Check sheet for the modelled part. Datum: model origin and axes. Units: mm. A direction names the side the tool comes from. Round coordinates to 2 decimals unless told otherwise and drop trailing zeros. Order: outer loops, then holes, each group sorted by start corner. A loop starts at its lowest first (then second) coordinate and runs counter-clockwise, first axis right, second up.
```python
from build123d import *

# Parameters (mm, degrees)
SKETCH2_R           = 4.826
CUT_EXTRUDE1_DEPTH  = 25.4
SKETCH3_W           = 14.986
SKETCH3_H           = 14.986
BOSS_EXTRUDE1_DEPTH = 12.7


with BuildPart() as part:
    # Sketch1 → Revolve1 (revolve)
    with BuildSketch(Plane.XY):
        Polygon((0, 0), (152.4, 0), (152.4, 12.7), (0, 15.875), align=None)
    revolve(axis=Axis((0, 0, 0), (1, 0, 0)))

    # Sketch2 → Cut-Extrude1 (cut)
    with BuildSketch(Plane(origin=(152.4, 0, 0), x_dir=(0, 0, -1), z_dir=(1, 0, 0))):
        Circle(SKETCH2_R)
    extrude(amount=-CUT_EXTRUDE1_DEPTH, mode=Mode.SUBTRACT)

    # Sketch3 → Boss-Extrude1 (add)
    with BuildSketch(Plane.ZY):
        Rectangle(SKETCH3_W, SKETCH3_H)
    extrude(amount=BOSS_EXTRUDE1_DEPTH)


solid = part.part
```
Item 1: Scan lines: line 1 along Y through (x, z) = (135, 0); line 2 along X through (y, z) = (-3, 0); line 3 along X through (y, z) = (-12, 3.5). Record each from-to range of solid material in increasing order.
Answer:
line 1: y = -13.06 to -4.83, 4.83 to 13.06
line 2: x = -12.7 to 127
line 3: x = 0 to 152.4
Item 2: Sectioned sample at C-C (x = 140.5). Record the cut outline in (y, z), and give its area (3 significant figures).
Answer:
outline: circle Ø25.9 at (0, 0); hole circle Ø9.65 at (0, 0)
area: 454 mm2
Item 3: Go/stop test with flat-tipped pins: P1, Ø10, axis at x = -7.5, y = -3.5, coming from the +Z side; P2, Ø12, axis at x = 49.5, y = -6.5, coming from the -Z side; P3, Ø5, axis at x = 10, z = -7, coming from the -Y side. Record where each tip stops, or that it passes through.
Answer:
P1: stops at z = 7.49
P2: stops at z = -14.86
P3: stops at y = -15.01
Item 4: Sectioned sample at D-D (x = 16). Record the cut outline in (y, z).
Answer:
outline: circle Ø31.08 at (0, 0)
Item 5: Release check for a two-part mould opening along Z. For faces 1 (the flat face through (-6, 0, -7.493)), 2 (the flat face through (-6, -7.493, 0)), 3 (the cylindrical face through (139.878, -2.937, 3.83)), 4 (the flat face through (127, 0, 0)) record: released by +Z, released by -Z, zero draft, split by the parting line, or undercut.
Answer:
face 1: released by -Z
face 2: zero draft
face 3: undercut
face 4: undercut
Item 6: Access from +Z, -Z, +X, -X, +Y, -Y to the whole of each face (thin tool, end or side, straight path). Record for faces 5 (the flat face through (-6, 7.493, 0)), 6 (the conical face through (75.133, -14.296, 0.629)), 7 (the flat face through (-6, 0, 7.493)).
Answer:
face 5: +Z, -Z, -X, +Y
face 6: +X
face 7: +Z, -X, +Y, -Y
Item 7: Sectioned sample at A-A (y = 0). Record the cut outline in (x, z) (3 decimals).
Answer:
outline: (-12.7, -7.493) - (0, -7.493) - (0, -15.875) - (152.4, -12.7) - (152.4, -4.826) - (127, -4.826) - (127, 4.826) - (152.4, 4.826) - (152.4, 12.7) - (0, 15.875) - (0, 7.493) - (-12.7, 7.493) - close
